The listing builds one solid part. Answer for the finished solid, in the listing's coordinates (mm). A direction names the side the tool comes from. Give positions to 0.01 mm unless a question says otherwise; leave off trailing zeros. Order: outer loops, then holes, each group sorted by start corner. A loop starts at its lowest first (then second) coordinate and runs counter-clockwise, first axis right, second up. Notation, with made-up numbers: (48, 48) - (90, 48) arc R8 ccw to (90, 57) - close; hole circle Ø1 at (-19.75, 58). An arc over 180 degrees is marked (long way). Use a Markdown table: item, result. Add a question column.
1) Straight lines are drawn through the part: line 1 (Y direction, x = 0, z = 2.25); line 2 (X direction, y = 0, z = 14). For each, find the intervals that lie inside material, in ascending order.
2) For faces 1 (the face through (0.867, 3.905, 12.605)), 2 (the face through (-10, 0, 7)), determine the directions among +Z, -Z, +X, -X, +Y, -Y from which every point of the face is accessible in a straight line to the end or side of a thin tool.
3) Find section B-B, the plane z = 4.25. Determine the outline of the cut face in (x, y).
4) Find section D-D, the plane z = 10.25. Determine the outline of the cut face in (x, y), plus the area to 3 significant figures.
5) Find section A-A, the plane y = 0. Determine the outline of the cut face in (x, z).
6) Flat-ended cylindrical pins translate along their axes: pin 1 (1.5 mm diameter, centred on x = 6, y = 5, fed in from +Z); pin 2 (3 mm diameter, centred on y = 7.5, z = 17, fed in from +X); pin 3 (1.5 mm diameter, centred on x = -2, y = -1, fed in from -Z); pin 4 (2.5 mm diameter, centred on x = -2, y = -0.5, fed in from +Z). Find the tip coordinate at first contact, or state that the pin passes through.
7) The mould has two halves that part along X. Classify faces 3 (the face through (0, -2, 2)), 4 (the face through (2, 1, 5)), 5 (the face through (-9.1, 9.14, 7.6)), 6 (the face through (0, 9, 18)): released by +X, released by -X, zero draft, split by the parting line, or undercut.
Autodesk Fusion 360 part; units mm, degrees
sketch "Sketch1" plane through (0, 0, 0) normal (0, 0, 1) x (1, 0, 0)
  line L0 (10, -10) -> (-10, -10)
  line L1 (-10, -10) -> (-10, 10)
  line L2 (-10, 10) -> (10, 10)
  line L3 (10, 10) -> (10, -10)
  line L4 (10, -10) -> (-10, 10) construction
  line L5 (-10, -10) -> (10, 10) construction
  dimension "d1" = 20
  dimension "d2" = 20
extrude "Extrude1" add sketch "Sketch1" along normal blind 20
sketch "Sketch2" plane through (0, 0, 20) normal (0, 0, 1) x (-1, 0, 0)
  line L0 (-10, -10) -> (10, -10)
  line L1 (10, -10) -> (10, 10)
  line L2 (10, 10) -> (-10, 10)
  line L3 (-10, 10) -> (-10, -10)
  circle A0 centre (0, 0) radius 2
  circle A1 centre (0, 0) radius 4
  dimension "d5" = 4
  dimension "d6" = 8
extrude "Extrude2" cut sketch "Sketch2" against normal blind 40 contours A0
extrude "Extrude3" cut sketch "Sketch2" against normal blind 17 contours A1
sketch "Sketch3" plane through (10, 0, 0) normal (1, 0, 0) x (0, 1, 0)
  line L0 (-10, 0) -> (10, 0)
  line L1 (10, 0) -> (10, 20)
  line L2 (10, 20) -> (-10, 20)
  line L3 (-10, 20) -> (-10, 0)
  circle A0 centre (0, 18) radius 3.5
  line L4 (0, 0) -> (0, 24.4173) construction
  dimension "d11" = 7
  dimension "d20" = 2
extrude "Extrude4" cut sketch "Sketch3" against normal blind 22 contours L2 A0 picked at (-0.83, 20.3844)
fillet "Fillet1" radius 5 6 edges at (10, -6.4361, 20) (0, -10, 20) (-10, -6.4361, 20) (-10, 6.4361, 20) (0, 10, 20) (10, 6.4361, 20)
fillet "Fillet2" radius 3 8 edges at (10, 10, 7.5) (8.5355, 8.5355, 18.5355) (10, -10, 7.5) (8.5355, -8.5355, 18.5355) (-10, 10, 7.5) (-8.5355, 8.5355, 18.5355) (-10, -10, 7.5) (-8.5355, -8.5355, 18.5355)
extrude "Extrude5" add 1 faces at (-3.311, 0.2981, 3) along direction (0, 0, 1) blind 2
The answers:
| question | item | result |
|---|---|---|
| 1 | line 1 | -10 to -2, 2 to 10 |
| 1 | line 2 | -10 to -4, 4 to 10 |
| 2 | face 1 | +Z |
| 2 | face 2 | +Z, -Z, -X, +Y, -Y |
| 3 | outline | (-10, -7) arc R3 ccw to (-7, -10) - (7, -10) arc R3 ccw to (10, -7) - (10, 7) arc R3 ccw to (7, 10) - (-7, 10) arc R3 ccw to (-10, 7) - close; hole circle Ø4 at (0, 0) |
| 4 | outline | (-10, -7) arc R3 ccw to (-7, -10) - (7, -10) arc R3 ccw to (10, -7) - (10, 7) arc R3 ccw to (7, 10) - (-7, 10) arc R3 ccw to (-10, 7) - close; hole circle Ø8 at (0, 0) |
| 4 | area | 342 mm2 |
| 5 | outline | (-10, 0) - (-2, 0) - (-2, 5) - (-4, 5) - (-4, 20) - (-5, 20) arc R5 ccw to (-10, 15) - close; (2, 0) - (10, 0) - (10, 15) arc R5 ccw to (5, 20) - (4, 20) - (4, 5) - (2, 5) - close |
| 6 | pin 1 | z = 19.99 |
| 6 | pin 2 | x = 9.97 |
| 6 | pin 3 | z = 0 |
| 6 | pin 4 | z = 5 |
| 7 | face 3 | undercut |
| 7 | face 4 | undercut |
| 7 | face 5 | released by -X |
| 7 | face 6 | zero draft |
